Can you work these out from the model? Positions are in its coordinate system, mm. Round coordinates to 2 decimals unless told otherwise and drop trailing zeros. Write each loop counter-clockwise with the first axis right and the second up, starting at its lowest first coordinate (ties: lowest second). Pieces come first, ordered by that corner, then holes. Notation, with made-up numbers: M -9.5,-21.5 L 29.5,-21.5 A22 cw 29.5,-6.5 Z; hole C -33.75,31.5 d6. An arc over 180 degrees is marked long. Answer as a JSON object with one key per item and string values. Group by question number.
1) I'm going to push flat-ended pins straight in: pin 1 Ø4 at (x, y) = (-64.07, 65.98) entering from +Z; pin 2 Ø2.5 at (x, y) = (20, -1.6) entering from -Z; pin 3 Ø4 at (x, z) = (-25.5, 5.5) entering from -Y; pin 4 Ø3.5 at (y, z) = (27, 5) entering from +X. Where does each tip first touch, or does it pass through?
2) Suppose I cut it at B-B, the plane z = 2.25. State how many separate pieces and enclosed holes the cut face has, and give its area (3 significant figures).
3) Suppose I cut it at D-D, the plane x = 68. Write out the boundary of the cut face in (y, z).
4) Suppose I cut it at A-A, the plane y = 29. Write out the boundary of the cut face in (x, z).
5) Suppose I cut it at C-C, the plane x = -69. Write out the boundary of the cut face in (y, z).
6) Please list where these lines run through material, in increasing order: L1, parallel to X at y = -1, z = 5.5; L2, parallel to Y at x = 6.5, z = 4.5; L3, parallel to Y at x = 63, z = 4.5. Write a range as [from, to].
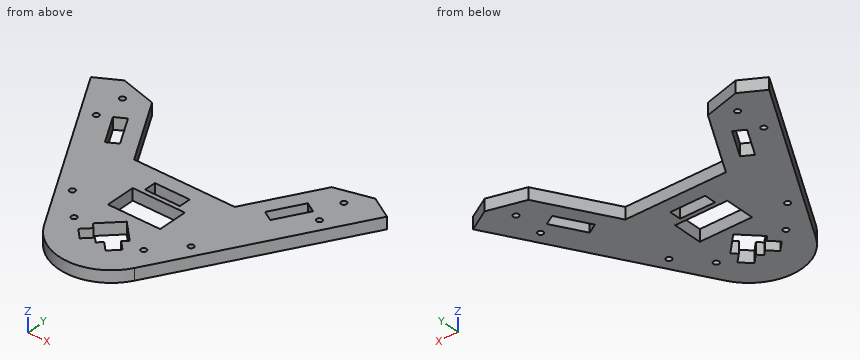
Autodesk Inventor part; units mm, degrees
ref_plane "YZ Plane" through (0, 0, 0) normal (1, 0, 0) x (0, 1, 0)
ref_plane "XZ Plane" through (0, 0, 0) normal (0, 1, 0) x (-1, 0, 0)
ref_plane "XY Plane" through (0, 0, 0) normal (0, 0, 1) x (1, 0, 0)
sketch "Sketch1" plane through (0, 0, 0) normal (0, 0, 1) x (1, 0, 0)
  line L0 (-10.6066, 0) -> (0, 10.6066)
  line L1 (0, 10.6066) -> (10.6066, 0)
  line L2 (10.6066, 0) -> (0, -10.6066)
  line L3 (0, -10.6066) -> (-10.6066, 0)
  arc A0 (-25.9808, -15) -> (25.9808, -15) centre (0, 0) ccw
  line L4 (25.9808, -15) -> (85, 87.2243)
  line L5 (10, 41.731) -> (10, 35)
  line L6 (10, 35) -> (-10, 35)
  line L7 (-10, 35) -> (-10, 41.731)
  line L8 (-10, 41.731) -> (10, 41.731)
  line L9 (-85, 87.2243) -> (-25.9808, -15)
  circle A1 centre (-49.0748, 40) radius 1.6
  circle A2 centre (-64.0748, 65.9808) radius 1.6
  circle A3 centre (49.0748, 40) radius 1.6
  circle A4 centre (64.0748, 65.9808) radius 1.6
  line L10 (-85, 87.2243) -> (-72.0096, 94.7243)
  line L11 (-51.5192, 89.2339) -> (-28.8675, 50)
  line L12 (-28.8675, 50) -> (28.8675, 50)
  line L13 (28.8675, 50) -> (51.5192, 89.2339)
  line L14 (2.6517, -7.955) -> (7.955, -2.6517)
  line L15 (7.955, -2.6517) -> (12.7145, -7.4112)
  line L16 (12.7145, -7.4112) -> (7.4112, -12.7145)
  line L17 (7.4112, -12.7145) -> (2.6517, -7.955)
  line L18 (-2.6517, -7.955) -> (-7.4112, -12.7145)
  line L19 (-7.4112, -12.7145) -> (-12.7145, -7.4112)
  line L20 (-12.7145, -7.4112) -> (-7.955, -2.6517)
  line L21 (-7.955, -2.6517) -> (-2.6517, -7.955)
  circle A5 centre (-38.567, 40) radius 1.6
  circle A6 centre (38.567, 40) radius 1.6
  circle A7 centre (-63.567, 83.3013) radius 1.6
  circle A8 centre (63.567, 83.3013) radius 1.6
  circle A9 centre (-20, -1.6) radius 1.6
  circle A10 centre (20, -1.6) radius 1.6
  line L22 (-57.4526, 69.5109) -> (-47.4526, 52.1904)
  line L23 (-47.4526, 52.1904) -> (-41.6234, 55.5559)
  line L24 (-41.6234, 55.5559) -> (-51.6234, 72.8764)
  line L25 (-51.6234, 72.8764) -> (-57.4526, 69.5109)
  line L26 (47.4526, 52.1904) -> (57.4526, 69.5109)
  line L27 (57.4526, 69.5109) -> (51.6234, 72.8764)
  line L28 (51.6234, 72.8764) -> (41.6234, 55.5559)
  line L29 (41.6234, 55.5559) -> (47.4526, 52.1904)
  line L30 (-15, 32.5) -> (15, 32.5)
  line L31 (15, 32.5) -> (15, 15.6066)
  line L32 (15, 15.6066) -> (-15, 15.6066)
  line L33 (-15, 15.6066) -> (-15, 32.5)
  line L34 (-10.6066, 0) -> (10.6066, 0)
  line L35 (25.9808, -15) -> (0, -60)
  line L36 (0, -60) -> (-25.9808, -15)
  line L37 (85, 87.2243) -> (72.0096, 94.7243)
  circle A11 centre (-34.0748, 14.0192) radius 1.6
  circle A12 centre (34.0748, 14.0192) radius 1.6
  line L38 (72.0096, 94.7243) -> (51.5192, 89.2339)
  line L39 (-51.5192, 89.2339) -> (-72.0096, 94.7243)
  point P0 (0, 0)
  point P1 (0, 35)
  point P2 (0, 32.5)
  dimension "d0" = 15
  dimension "d9" = 30
  dimension "d11" = 6.731
  dimension "d12" = 20
  dimension "d25" = 60
  dimension "d34" = 3.2
  dimension "d36" = 30
  dimension "d38" = 30
  dimension "d40" = 7.5
  dimension "d41" = 7.5
  dimension "d42" = 7.5
  dimension "d43" = 7.5
  dimension "d45" = 40
  dimension "d54" = 50
  dimension "d55" = 0
  dimension "d56" = 0
  dimension "d57" = 7.5
  dimension "d58" = 3.75
  dimension "d63" = 15
  dimension "d64" = 3.2
  dimension "d66" = 50
  dimension "d67" = 15
  dimension "d68" = 15
  dimension "d73" = 20
  dimension "d74" = 15
  dimension "d75" = 15
  dimension "d76" = 15
  dimension "d77" = 15
  dimension "d79" = 35
  dimension "d80" = 2.5
  dimension "d81" = 5
  dimension "d82" = 30
  dimension "d83" = 20
  dimension "d84" = 20
  dimension "d85" = 40
  dimension "d86" = 170
  dimension "d88" = 30
  dimension "d89" = 30
  dimension "d90" = 7.5
  dimension "d91" = 7.5
  dimension "d92" = 135
  dimension "d93" = 30
  dimension "d94" = 45
  dimension "d95" = 15
extrude "Extrusion2" add sketch "Sketch1" along normal blind 6.731 contours L9 L10 L39 L11 L12 L13 L38 L37 L4 A0 | A5 | A6
sketch "Sketch2" plane through (0, 0, 6.731) normal (0, 0, 1) x (1, 0, 0)
  circle A0 centre (49.0748, 40) radius 1.6
  circle A1 centre (-49.0748, 40) radius 1.6
extrude "Extrusion3" add sketch "Sketch2" against normal up to surface (6.731 mm away)
equation "\"d38\" = d36"
equation "\"d41\" = d40"
equation "\"d58\" = 0.5 * d57"
equation "\"THICKA\" = 3.175"
equation "\"THICKB\" = 6.731"
equation "\"THICKC\" = 12.7"
equation "\"BALLDIA\" = 12"
equation "\"MAGDIA\" = 9.5"
equation "\"THICKPLY\" = 5"
properties part number "Frame_Upper_Plate_Bottom"
Results:
{
 "1": {"pin 1": "z = 6.73", "pin 2": "through", "pin 3": "y = -18.65", "pin 4": "x = 51.24"},
 "2": {"separate pieces": "1", "enclosed holes": "13", "area": "7,940 mm^2"},
 "3": {"outline": "M 57.78,0 L 93.65,0 L 93.65,6.73 L 57.78,6.73 Z"},
 "4": {"outline": "M -51.38,0 L -15,0 L -15,6.73 L -51.38,6.73 Z; M 15,0 L 51.38,0 L 51.38,6.73 L 15,6.73 Z"},
 "5": {"outline": "M 59.51,0 L 93.92,0 L 93.92,6.73 L 59.51,6.73 Z"},
 "6": {"L1": "[-34.06, -21.48], [-18.52, -9.61], [9.61, 18.52], [21.48, 34.06]", "L2": "[-29.29, -11.8], [4.11, 15.61], [32.5, 35], [41.73, 50]", "L3": "[49.12, 64.8], [67.17, 81.81], [84.8, 92.31]"}
}
